Autodesk Inventor part; units mm, degrees
ref_plane "YZ Plane" through (0, 0, 0) normal (1, 0, 0) x (0, 1, 0)
ref_plane "XZ Plane" through (0, 0, 0) normal (0, 1, 0) x (-1, 0, 0)
ref_plane "XY Plane" through (0, 0, 0) normal (0, 0, 1) x (1, 0, 0)
sketch "Sketch1" plane through (0, 0, 0) normal (0, 0, 1) x (1, 0, 0)
  arc A0 (0, 4.9998) -> (-5, -0.0002) centre (0, -0.0002) ccw
  arc A1 (-6, -5.028) -> (-5, -4.028) centre (-6, -4.028) ccw
  line L0 (0, -5.5) -> (-6, -5.5)
  line L1 (-6, -5.5) -> (-6, -5.028)
  line L2 (-5, -0.0002) -> (-5, -4.028)
  arc A2 (0, 3.4998) -> (-3.5, -0.0002) centre (0, -0.0002) ccw
  line L3 (-3.5, -0.0002) -> (-3.5, -5.5)
  line L4 (0, 4.9998) -> (0, -5.5)
  point P0 (0, 0)
  dimension "d7" = 90
  dimension "d9" = 6
  dimension "d13" = 1
  dimension "d16" = 10.4998
  dimension "d17" = 5
  dimension "d18" = 3.5
  dimension "d19" = 90
  dimension "d21" = 5.5
  dimension "d22" = 5
  dimension "d23" = 3.5
revolve "Revolution1" add sketch "Sketch1" angle 360 about axis through (0, 4.9998, 0) along (0, -1, 0) contours L4 A2 L3 L0 L1 A1 L2 A0
sketch "Sketch2" plane through (0, 0, 0) normal (0, 1, 0) x (-1, 0, 0)
  point P0 (0, 0)
sketch "Sketch3" plane through (0, 0, 0) normal (0, 1, 0) x (-1, 0, 0)
  circle A0 centre (0, 0) radius 0.75
  dimension "d25" = 1.5
extrude "Extrusion1" cut sketch "Sketch3" along normal up to surface
sketch "Sketch4" plane through (0, 0, 0) normal (1, 0, 0) x (0, 1, 0)
  line L0 (-5.5, -6) -> (-5.5, 6)
  line L1 (5.5, -0.375) -> (-5.5, -0.375)
  line L2 (-5.5, -0.375) -> (-5.5, 0.375)
  line L3 (-5.5, 0.375) -> (5.5, 0.375)
  line L4 (5.5, 0.375) -> (5.5, -0.375)
  line L5 (5.5, -0.375) -> (-5.5, 0.375) construction
  line L6 (-5.5, -0.375) -> (5.5, 0.375) construction
  point P0 (0, 0)
  dimension "d28" = 0.75
extrude "Extrusion2" cut sketch "Sketch4" along normal up to surface
properties part number "Puller"
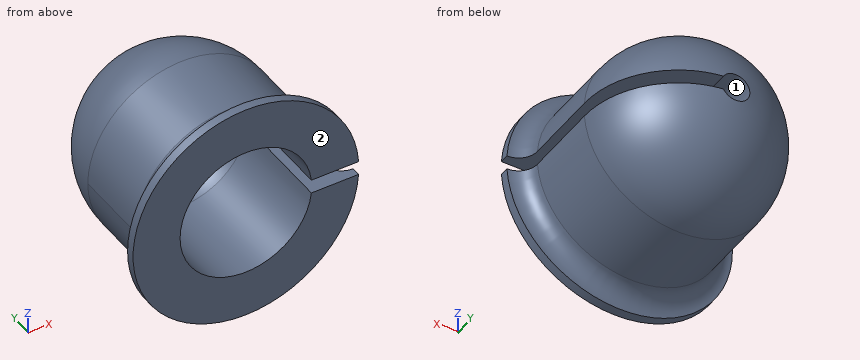
Geometry: final body of the model. Coordinates: model frame, mm. Face numbers are marked on the shaded views. Give positions to 0.01 mm unless a question says otherwise; leave off trailing zeros. Write each loop counter-clockwise with the first axis right and the second up, starting at its lowest first coordinate (ties: lowest second). Pieces come first, ordered by that corner, then holes.
1. Line query: probe 1 along X at (y, z) = (0.75, 0.75); probe 2 along Z at (x, y) = (-2.75, -4.5); probe 3 along Z at (x, y) = (2.25, 3.5) (3 decimals). Output: solid intervals per line, ascending.
2. Section query A-A, the plane x = 0. Return loops of the section in (y, z), then the cut area to 3 significant figures.
3. Draft query along X for the marked faces 1 and 2. Return one class per face: released by +X, released by -X, zero draft, split by the parting line, or undercut.
4. Pin query (flat end, axial travel): P1, Ø3, axis at x = 0.5, z = 3, coming from the +Y side; P2, Ø1.6, axis at x = 2.5, y = 0.5, coming from the -Z side; P3, Ø4, axis at x = 0, y = -1, coming from the +Z side. Return the tip coordinate at first contact, or that it passes through.
5. Section query C-C, the plane y = 1.25. Return loops of the section in (x, z) (3 decimals).
6. Section query B-B, the plane y = -3.5. Return loops of the section in (x, z) (3 decimals).
Computed:
1. probe 1: x = -4.89 to -3.34, 3.34 to 4.89
1. probe 2: z = -4.32 to -2.17, 2.17 to 4.32
1. probe 3: z = -2.772 to -0.375, 0.375 to 2.772
2. outline: (-5.5, -6) - (-5.03, -6) arc R1 cw to (-4.03, -5) - (0, -5) arc R5 ccw to (4.94, -0.75) - (3.42, -0.75) arc R3.5 cw to (0, -3.5) - (-5.5, -3.5) - close; (-5.5, 3.5) - (0, 3.5) arc R3.5 cw to (3.42, 0.75) - (4.94, 0.75) arc R5 ccw to (0, 5) - (-4.03, 5) arc R1 cw to (-5.03, 6) - (-5.5, 6) - close
2. area: 35.6 mm2
3. face 1: undercut
3. face 2: zero draft
4. P1: stops at y = 4.76
4. P2: stops at z = -4.68
4. P3: stops at z = 5
5. outline: (3.248, -0.375) arc R3.269 cw (long way) to (3.248, 0.375) - (4.827, 0.375) arc R4.841 ccw (long way) to (4.827, -0.375) - close
6. outline: (3.48, -0.375) arc R3.5 cw (long way) to (3.48, 0.375) - (4.986, 0.375) arc R5 ccw (long way) to (4.986, -0.375) - close
